from build123d import *

# Parameters (mm, degrees)
F0_W     = 6
F0_H     = 80
F1_DEPTH = 3
F2_R     = 1.5
F3_DEPTH = 1.5
F4_R     = 1.5
F5_DEPTH = 45


with BuildPart() as f1:
    # F0 (on Front) → F1 (new body)
    with BuildSketch(Plane.XZ):
        Rectangle(F0_W, F0_H)
    extrude(amount=F1_DEPTH)

    # F2 (on face) → F3 (cut)
    with BuildSketch(Plane.XZ.offset(3)):
        with Locations((0, -20)):
            Circle(F2_R)
    extrude(amount=-F3_DEPTH, mode=Mode.SUBTRACT)

    # F4 (on face) → F5 (join)
    with BuildSketch(Plane.XZ.offset(3)):
        with Locations((0, 10)):
            Circle(F4_R)
        with Locations((0, 30)):
            Circle(F4_R)
    extrude(amount=F5_DEPTH)


solid = f1.part
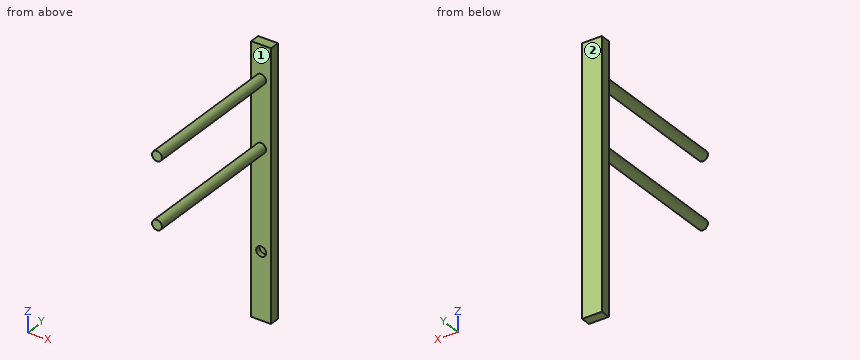
Geometry check sheet. Reference: the model listing, model coordinates, mm. Face numbers are marked on the shaded views. Round coordinates to 2 decimals unless told otherwise and drop trailing zeros. Order: outer loops, then holes, each group sorted by start corner. A loop starts at its lowest first (then second) coordinate and runs counter-clockwise, first axis right, second up. Notation, with made-up numbers: M 46.5,-12.5 L 90.5,-12.5 A23 cw 90.5,8.5 Z; hole C 53,34.5 d6. An arc over 180 degrees is marked long. Answer in a Markdown table with one row per item.
(1) Sectioned sample at A-A, the plane z = 10. Record the cut outline in (x, y), and give its area (3 significant figures).
Responses:
| item | result |
|---|---|
| outline | M -3,-3 L -1.5,-3 L -1.5,-48 L 1.5,-48 L 1.5,-3 L 3,-3 L 3,0 L -3,0 Z |
| area | 153 mm² |
(2) Sectioned sample at C-C, the plane y = -19. Record the cut outline in (x, z), and give its area (3 significant figures).
Responses:
| item | result |
|---|---|
| outline | C 0,10 d3; C 0,30 d3 |
| area | 14.1 mm² |
(3) Sectioned sample at B-B, the plane x = 0. Record the cut outline in (y, z).
Responses:
| item | result |
|---|---|
| outline | M -48,8.5 L -3,8.5 L -3,-18.5 L -1.5,-18.5 L -1.5,-21.5 L -3,-21.5 L -3,-40 L 0,-40 L 0,40 L -3,40 L -3,31.5 L -48,31.5 L -48,28.5 L -3,28.5 L -3,11.5 L -48,11.5 Z |
(4) Go/stop test with flat-tipped pins: P1, Ø1, axis at x = -1.5, y = -27.5, coming from the +Z side; P2, Ø1.5, axis at x = -0.5, z = -19.5, coming from the -Y side. Record where each tip stops, or that it passes through.
Responses:
| item | result |
|---|---|
| P1 | stops at z = 31.12 |
| P2 | stops at y = -1.5 |
(5) Sectioned sample at D-D, the plane z = -20. Record the cut outline in (x, y).
Responses:
| item | result |
|---|---|
| outline | M -3,-3 L -1.5,-3 L -1.5,-1.5 L 1.5,-1.5 L 1.5,-3 L 3,-3 L 3,0 L -3,0 Z |
(6) Draft check along Z on the marked faces 1 and 2. Enter one of: released by +Z, released by -Z, zero draft, split by the parting line, or undercut.
Responses:
| item | result |
|---|---|
| face 1 | undercut |
| face 2 | zero draft |
(7) Scan lines: probe 1 along Z at (x, y) = (0, -1.75); probe 2 along Y at (x, z) = (1.95, -9); probe 3 along Z at (x, y) = (-0.3, -18.5). Record each from-to range of solid material in increasing order. Write a range as from..to.
Responses:
| item | result |
|---|---|
| probe 1 | z = -40..-21.5, -18.5..40 |
| probe 2 | y = -3..0 |
| probe 3 | z = 8.53..11.47, 28.53..31.47 |
